Source: three-view drawing plus pictorial views. Frame: mm from the lowest corner of the part. A direction names the side the tool comes from. Give positions to 0.01 mm unless a question says otherwise; leave off trailing zeros. Loops run counter-clockwise (first coordinate to the right, second up) from the corner with the lowest first, then second, coordinate; pieces in that order, holes last. Notation, with made-up numbers: (43.5, 29.5) -> (94.5, 29.5) arc R10 cw to (94.5, 34.5) -> close; hole circle Ø6 at (55.25, 2). An arc over 180 degrees is marked (long way). Put each result on its own line as item: value.
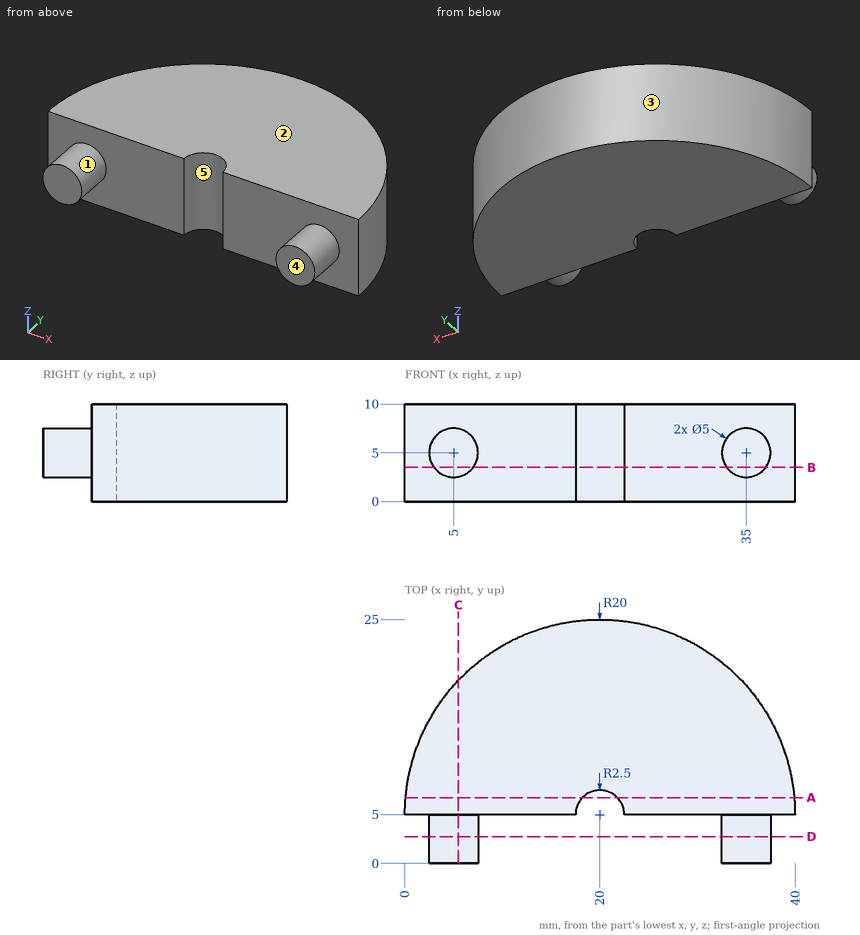
(1) Reachability of the marked faces 1 and 2 from +Z, -Z, +X, -X, +Y, -Y: full face, straight path, thin tool, end or side. Return the list, or none.
Calculated:
face 1: -Y
face 2: +Z, +X, -X, +Y, -Y
(2) Line query: probe 1 along X at (y, z) = (2.25, 7.25); probe 2 along X at (y, z) = (4.5, 4.5); probe 3 along X at (y, z) = (17.5, 1.25). Output: solid intervals per line, ascending. Write a range as from..to.
Calculated:
probe 1: x = 3.91..6.09, 33.91..36.09
probe 2: x = 2.55..7.45, 32.55..37.45
probe 3: x = 4.39..35.61
(3) Section A-A on y = 6.75. Return loops of the section in (x, z).
Calculated:
outline: (0.08, 0) -> (18.21, 0) -> (18.21, 10) -> (0.08, 10) -> close; (21.79, 0) -> (39.92, 0) -> (39.92, 10) -> (21.79, 10) -> close
(4) Section D-D on y = 2.75. Return loops of the section in (x, z), then the cut area to 3 significant figures.
Calculated:
outline: circle Ø5 at (5, 5); circle Ø5 at (35, 5)
area: 39.3 mm²
(5) Draft query along X for the marked faces 3, 4 and 5. Return one class per face: released by +X, released by -X, zero draft, split by the parting line, or undercut.
Calculated:
face 3: split by the parting line
face 4: zero draft
face 5: undercut
(6) First-contact query: P1, Ø4, axis at y = 12.5, z = 4, coming from the +X side; P2, Ø3, axis at x = 10, z = 5, coming from the -Y side; P3, Ø3, axis at y = 3, z = 5, coming from the +X side. Flat tips, straight axial feed; report the tip coordinate or a pass-through.
Calculated:
P1: stops at x = 39.23
P2: stops at y = 5
P3: stops at x = 37.5
(7) Section B-B on z = 3.5. Return loops of the section in (x, y).
Calculated:
outline: (0, 5) -> (3, 5) -> (3, 0) -> (7, 0) -> (7, 5) -> (17.5, 5) arc R2.5 cw to (22.5, 5) -> (33, 5) -> (33, 0) -> (37, 0) -> (37, 5) -> (40, 5) arc R20 ccw to start
(8) Section C-C on x = 5.5. Return loops of the section in (y, z).
Calculated:
outline: (0, 2.55) -> (5, 2.55) -> (5, 0) -> (18.77, 0) -> (18.77, 10) -> (5, 10) -> (5, 7.45) -> (0, 7.45) -> close
